Work out the finished part from the listing and answer in its coordinate system (mm). A direction names the side the tool comes from. Coordinates: 2 decimals unless noted, no trailing zeros. Loops run counter-clockwise (first coordinate to the right, second up) from the corner with the lowest first, then second, coordinate; pieces in that order, holes last. Notation, with made-up numbers: (46.5, 12.5) - (55.5, 12.5) arc R13 ccw to (55.5, 22.5) - close; hole circle Ø7 at (-5, -26). An arc over 180 degrees is marked (long way). Write each question's results on one line, items separated by ' | '. Start each with the question number.
1. Find the intervals of material crossed by line 1 along X through (y, z) = (-1.25, 0) (3 decimals); line 2 along Z through (x, y) = (61, 3.5); line 3 along Z through (x, y) = (-75.5, 1.75), in increasing order. Write a range as [from, to].
2. A cutting plane is placed at D-D on z = 0. State how many separate pieces and enclosed holes the cut face has, then the cut area to 3 significant figures.
3. A cutting plane is placed at B-B on x = -52. Determine the outline of the cut face in (y, z), then the cut area to 3 significant figures.
4. A cutting plane is placed at C-C on x = -92. Determine the outline of the cut face in (y, z) (3 decimals).
5. Determine the mould class of faces 4 (the cylindrical face through (30.04, 0.06, 95.38)), 5 (the flat face through (62.23, 4.5, -31.31)), 6 (the cylindrical face through (-88.85, -0.06, -0.41)) for opening direction Z: released by +Z, released by -Z, zero draft, split by the parting line, or undercut.
6. A cutting plane is placed at A-A on z = -77.5. Determine the outline of the cut face in (x, y) (1 decimal), then the cut area to 3 significant figures.
7. Each of these flat-tipped pins is pushed along its axis until it touches: P1, Ø10, axis at x = -92, z = 0, coming from the -Y side; P2, Ø4, axis at y = 1, z = -34, coming from the -X side; P3, Ø5, axis at x = -29.5, y = -2, coming from the +Z side; P4, Ø2, axis at y = -2, z = -76, coming from the +X side. Where does it stop, or does it pass through?
8. Which of the six approach directions +Z, -Z, +X, -X, +Y, -Y give full straight-line access (tool end or side, diameter ignored) to faces 1 (the cylindrical face through (82.77, -3.02, -10.87)), 2 (the cylindrical face through (0.95, -0.06, -74.47)), 3 (the flat face through (45, 1.588, -70.5))?
from build123d import *

# Parameters (mm, degrees)
SKETCH1_R             = 100
SKETCH1_R_2           = 3.175
SKETCH1_R_3           = 86.02
BOSS_EXTRUDE1_DEPTH   = 4.5
SKETCH1_R_4           = 83.48
SKETCH1_R_5           = 69.5
BOSS_EXTRUDE1_2_DEPTH = 4.5
SKETCH1_3_R           = 86.02
SKETCH1_3_R_2         = 83.48
BOSS_EXTRUDE2_DEPTH   = 1.5875


with BuildPart() as part:
    # Sketch1 → Boss-Extrude1 (new, symmetric)
    with BuildSketch(Plane(origin=(0, 0, 0), x_dir=(1, 0, 0), z_dir=(0, 1, 0))):
        with Locations(Location((0, 0, 0), (0, 0, 270))):
            Circle(SKETCH1_R)
        with Locations(Location((-92, 0, 0), (0, 0, 270))):
            Circle(SKETCH1_R_2, mode=Mode.SUBTRACT)
        with Locations(Location((92, 0, 0), (0, 0, 270))):
            Circle(SKETCH1_R_2, mode=Mode.SUBTRACT)
        with Locations(Location((0, 0, 0), (0, 0, 270))):
            Circle(SKETCH1_R_3, mode=Mode.SUBTRACT)
        with Locations(Location((0, -92, 0), (0, 0, 270))):
            Circle(SKETCH1_R_2, mode=Mode.SUBTRACT)
        with Locations(Location((0, 92, 0), (0, 0, 270))):
            Circle(SKETCH1_R_2, mode=Mode.SUBTRACT)
    extrude(amount=BOSS_EXTRUDE1_DEPTH, both=True)



with BuildPart() as body_2:
    # Sketch1 → Boss-Extrude1 2 (new, symmetric)
    with BuildSketch(Plane(origin=(0, 0, 0), x_dir=(1, 0, 0), z_dir=(0, 1, 0))):
        with Locations(Location((0, 0, 0), (0, 0, 270))):
            Circle(SKETCH1_R_4)
        with Locations(Location((0, 77.5, 0), (0, 0, 270))):
            Circle(SKETCH1_R_2, mode=Mode.SUBTRACT)
        with Locations(Location((-77.5, 0, 0), (0, 0, 270))):
            Circle(SKETCH1_R_2, mode=Mode.SUBTRACT)
        with Locations(Location((0, -77.5, 0), (0, 0, 270))):
            Circle(SKETCH1_R_2, mode=Mode.SUBTRACT)
        with Locations(Location((77.5, 0, 0), (0, 0, 270))):
            Circle(SKETCH1_R_2, mode=Mode.SUBTRACT)
        with Locations(Location((0, 0, 0), (0, 0, 270))):
            Circle(SKETCH1_R_5, mode=Mode.SUBTRACT)
    extrude(amount=BOSS_EXTRUDE1_2_DEPTH, both=True)


with BuildPart() as part_1:
    add(part.part)

    add(body_2.part)  # Boss-Extrude2 merges body 2
    # Sketch1_3 → Boss-Extrude2 (add, symmetric)
    with BuildSketch(Plane(origin=(0, 0, 0), x_dir=(1, 0, 0), z_dir=(0, 1, 0))):
        with Locations(Location((0, 0, 0), (0, 0, 270))):
            Circle(SKETCH1_3_R)
        with Locations(Location((0, 0, 0), (0, 0, 270))):
            Circle(SKETCH1_3_R_2, mode=Mode.SUBTRACT)
    extrude(amount=BOSS_EXTRUDE2_DEPTH, both=True)


solid = part_1.part
Values:
1) line 1: [-100, -95.175], [-88.825, -80.675], [-74.325, -69.5], [69.5, 74.325], [80.675, 88.825], [95.175, 100] | line 2: [-79.24, -60.65], [-56.99, -33.31], [33.31, 56.99], [60.65, 79.24] | line 3: [-65.57, -41.22], [-35.62, -2.47], [2.47, 35.62], [41.22, 65.57]
2) separate pieces: 6 | enclosed holes: 0 | area: 291 mm^2
3) outline: (-4.5, -85.42) - (4.5, -85.42) - (4.5, -68.52) - (1.59, -68.52) - (1.59, -65.31) - (4.5, -65.31) - (4.5, -46.11) - (-4.5, -46.11) - (-4.5, -65.31) - (-1.59, -65.31) - (-1.59, -68.52) - (-4.5, -68.52) - close; (-4.5, 46.11) - (4.5, 46.11) - (4.5, 65.31) - (1.59, 65.31) - (1.59, 68.52) - (4.5, 68.52) - (4.5, 85.42) - (-4.5, 85.42) - (-4.5, 68.52) - (-1.59, 68.52) - (-1.59, 65.31) - (-4.5, 65.31) - close | area: 670 mm^2
4) outline: (-4.5, -39.192) - (4.5, -39.192) - (4.5, -3.175) - (-4.5, -3.175) - close; (-4.5, 3.175) - (4.5, 3.175) - (4.5, 39.192) - (-4.5, 39.192) - close
5) face 4: split by the parting line | face 5: zero draft | face 6: undercut
6) outline: (-63.2, -4.5) - (-37.3, -4.5) - (-37.3, -1.6) - (-31, -1.6) - (-31, -4.5) - (-3.2, -4.5) - (-3.2, 4.5) - (-31, 4.5) - (-31, 1.6) - (-37.3, 1.6) - (-37.3, 4.5) - (-63.2, 4.5) - close; (3.2, -4.5) - (31, -4.5) - (31, -1.6) - (37.3, -1.6) - (37.3, -4.5) - (63.2, -4.5) - (63.2, 4.5) - (37.3, 4.5) - (37.3, 1.6) - (31, 1.6) - (31, 4.5) - (3.2, 4.5) - close | area: 1,010 mm^2
7) P1: y = -4.5 | P2: x = -94.74 | P3: z = 96.29 | P4: x = 66.14
8) face 1: -Y | face 2: +Y, -Y | face 3: +Y
